Part print with two shaded views. Sizes in mm from the minimum x, y, z corner. Round coordinates to 2 decimals unless told otherwise and drop trailing zeros. Write each loop counter-clockwise with the first axis right and the second up, starting at its lowest first coordinate (ties: lowest second). Pieces come first, ordered by that corner, then holes. Notation, with made-up numbers: (14.5, 38.5) -> (63.5, 38.5) arc R20 cw to (63.5, 54.5) -> close; hole circle Ø4 at (80.5, -37.75). An arc over 180 degrees is marked (long way). Answer in a Markdown table with one row per item.
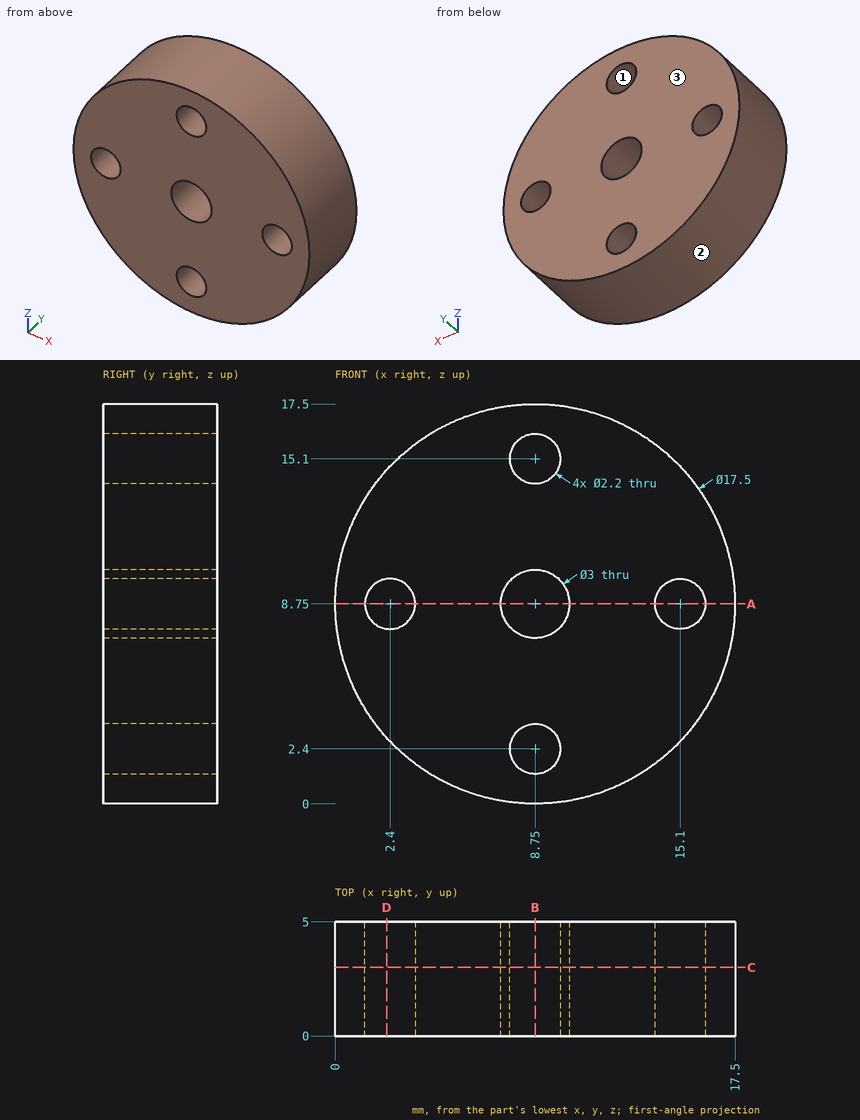
Q1. Wall check: line 1 (Z direction, x = 8.75, y = 1.45); line 2 (X direction, y = 2.85, z = 9.5). Give the ranges that are in metal, low to high. Write a range as [from, to].
A:
| item | result |
|---|---|
| line 1 | [0, 1.3], [3.5, 7.25], [10.25, 14], [16.2, 17.5] |
| line 2 | [0.03, 1.6], [3.2, 7.45], [10.05, 14.3], [15.9, 17.47] |
Q2. Saw through at D-D on x = 2.25. Write the cut outline in (y, z), plus the area to 3 significant figures.
A:
| item | result |
|---|---|
| outline | (0, 2.89) -> (5, 2.89) -> (5, 7.66) -> (0, 7.66) -> close; (0, 9.84) -> (5, 9.84) -> (5, 14.61) -> (0, 14.61) -> close |
| area | 47.7 mm² |
Q3. Saw through at B-B on x = 8.75. Write the cut outline in (y, z).
A:
| item | result |
|---|---|
| outline | (0, 0) -> (5, 0) -> (5, 1.3) -> (0, 1.3) -> close; (0, 3.5) -> (5, 3.5) -> (5, 7.25) -> (0, 7.25) -> close; (0, 10.25) -> (5, 10.25) -> (5, 14) -> (0, 14) -> close; (0, 16.2) -> (5, 16.2) -> (5, 17.5) -> (0, 17.5) -> close |
Q4. Two-plate mould, pull along X, no slides. Class the marked faces 1, 2 and 3: released by +X, released by -X, zero draft, split by the parting line, or undercut.
A:
| item | result |
|---|---|
| face 1 | undercut |
| face 2 | split by the parting line |
| face 3 | zero draft |
Q5. Drop a flat-ended pin along its axis: P1, Ø1, axis at x = 4.5, y = 1.5, coming from the -Z side. Give the stop position or say it passes through.
A:
| item | result |
|---|---|
| P1 | z = 0.84 |
Q6. Saw through at C-C on y = 3. Write the cut outline in (x, z), plus the area to 3 significant figures.
A:
| item | result |
|---|---|
| outline | circle Ø17.5 at (8.75, 8.75); hole circle Ø2.2 at (2.4, 8.75); hole circle Ø3 at (8.75, 8.75); hole circle Ø2.2 at (8.75, 2.4); hole circle Ø2.2 at (8.75, 15.1); hole circle Ø2.2 at (15.1, 8.75) |
| area | 218 mm² |
Q7. Saw through at A-A on z = 8.75. Write the cut outline in (x, y), plus the area to 3 significant figures.
A:
| item | result |
|---|---|
| outline | (0, 0) -> (1.3, 0) -> (1.3, 5) -> (0, 5) -> close; (3.5, 0) -> (7.25, 0) -> (7.25, 5) -> (3.5, 5) -> close; (10.25, 0) -> (14, 0) -> (14, 5) -> (10.25, 5) -> close; (16.2, 0) -> (17.5, 0) -> (17.5, 5) -> (16.2, 5) -> close |
| area | 50.5 mm² |
